Autodesk Inventor part; units mm, degrees
ref_plane "YZ Plane" through (0, 0, 0) normal (1, 0, 0) x (0, 1, 0)
ref_plane "XZ Plane" through (0, 0, 0) normal (0, 1, 0) x (-1, 0, 0)
ref_plane "XY Plane" through (0, 0, 0) normal (0, 0, 1) x (1, 0, 0)
sketch "Náčrt1" plane through (0, 0, 0) normal (0, 0, 1) x (1, 0, 0)
  line L0 (7.0986, 0.1592) -> (11.0986, 0.1592)
  line L1 (11.0986, 0.1592) -> (11.0986, 6.6592)
  line L2 (11.0986, 6.6592) -> (17.6486, 6.6592)
  line L3 (17.6486, 6.6592) -> (17.6486, 0.1592)
  line L4 (17.6486, 0.1592) -> (21.6486, 0.1592)
  line L5 (21.6486, 0.1592) -> (21.6486, 13.1592)
  line L6 (21.6486, 13.1592) -> (7.0986, 13.1592)
  line L7 (7.0986, 13.1592) -> (7.0986, 0.1592)
  point P0 (0, 0)
  dimension "d0" = 6.55
  dimension "d1" = 4
  dimension "d2" = 4
  dimension "d3" = 6.5
  dimension "d4" = 13
extrude "Vysunutí1" add sketch "Náčrt1" along normal blind 5.95
equation "\"d2\" = d1"
properties part number "Spacer"
The model under review builds one solid part; all positions refer to its coordinate system, in mm. A direction names the side the tool comes from. Coordinates: 2 decimals unless noted, no trailing zeros. Write each loop counter-clockwise with the first axis right and the second up, starting at its lowest first coordinate (ties: lowest second). Pieces come first, ordered by that corner, then holes. Notation, with made-up numbers: (4.25, -25) -> (53.25, -25) arc R13 ccw to (53.25, -2) -> close; hole circle Ø3 at (6.5, 72.25). An arc over 180 degrees is marked (long way). One line per item, written item: value. Start each with the question number.
Q1. To check wall thickness, follow probe 1 along X at (y, z) = (1, 1.3); probe 2 along Y at (x, z) = (14.25, 3.05). State the ranges of each line that lie inside material, in increasing order.
Q2. For faces 1 (the face through (11.099, 3, 3)), 2 (the face through (14, 8, 0)), list the 3-axis set-ups (+Z, -Z, +X, -X, +Y, -Y) from which the entire face can be reached by the end or side of a thin tool; tool diameter is ignored.
Q3. Add section A-A, the plane y = 4.5. Give the boundary of the cut face in (x, z).
Q4. Add section B-B, the plane z = 5.25. Give the boundary of the cut face in (x, y).
Q5. Clearance check with a flat-ended pin moving along its axis: P1, Ø1.8, axis at x = 13, z = 2, coming from the -Y side. State where the tip first meets the part, or that it passes through.
Q6. The part is to be moulded in two halves that separate along X. For faces 3 (the face through (14, 8, 5.95)), 4 (the face through (17.649, 3, 3)), 5 (the face through (7.099, 7, 3)), say which applies: +X half, -X half, draft (parallel to the pull), parting line (faces both ways), or undercut.
Q7. Add section C-C, the plane x = 13.25. Give the boundary of the cut face in (y, z).
Response:
1. probe 1: 7.1 to 11.1, 17.65 to 21.65
1. probe 2: 6.66 to 13.16
2. face 1: +Z, -Z, -Y
2. face 2: -Z, +X, -X, +Y, -Y
3. outline: (7.1, 0) -> (11.1, 0) -> (11.1, 5.95) -> (7.1, 5.95) -> close; (17.65, 0) -> (21.65, 0) -> (21.65, 5.95) -> (17.65, 5.95) -> close
4. outline: (7.1, 0.16) -> (11.1, 0.16) -> (11.1, 6.66) -> (17.65, 6.66) -> (17.65, 0.16) -> (21.65, 0.16) -> (21.65, 13.16) -> (7.1, 13.16) -> close
5. P1: y = 6.66
6. face 3: draft
6. face 4: undercut
6. face 5: -X half
7. outline: (6.66, 0) -> (13.16, 0) -> (13.16, 5.95) -> (6.66, 5.95) -> close
